Could you check a few things on this drawing? It's one solid part, dimensions in mm from its lowest x, y, z. A direction names the side the tool comes from. Give positions to 0.01 mm unless a question says otherwise; leave off trailing zeros. Order: outer loops, then holes, each group sorted by start corner. A loop starts at its lowest first (then second) coordinate and runs counter-clockwise, first axis right, second up. Notation, with made-up numbers: (52, 75.5) - (106, 75.5) arc R26 ccw to (106, 98.5) - close; hole circle Ø7 at (32.5, -26.75). An arc over 180 degrees is marked (long way). Answer as CSV lines item,"result".
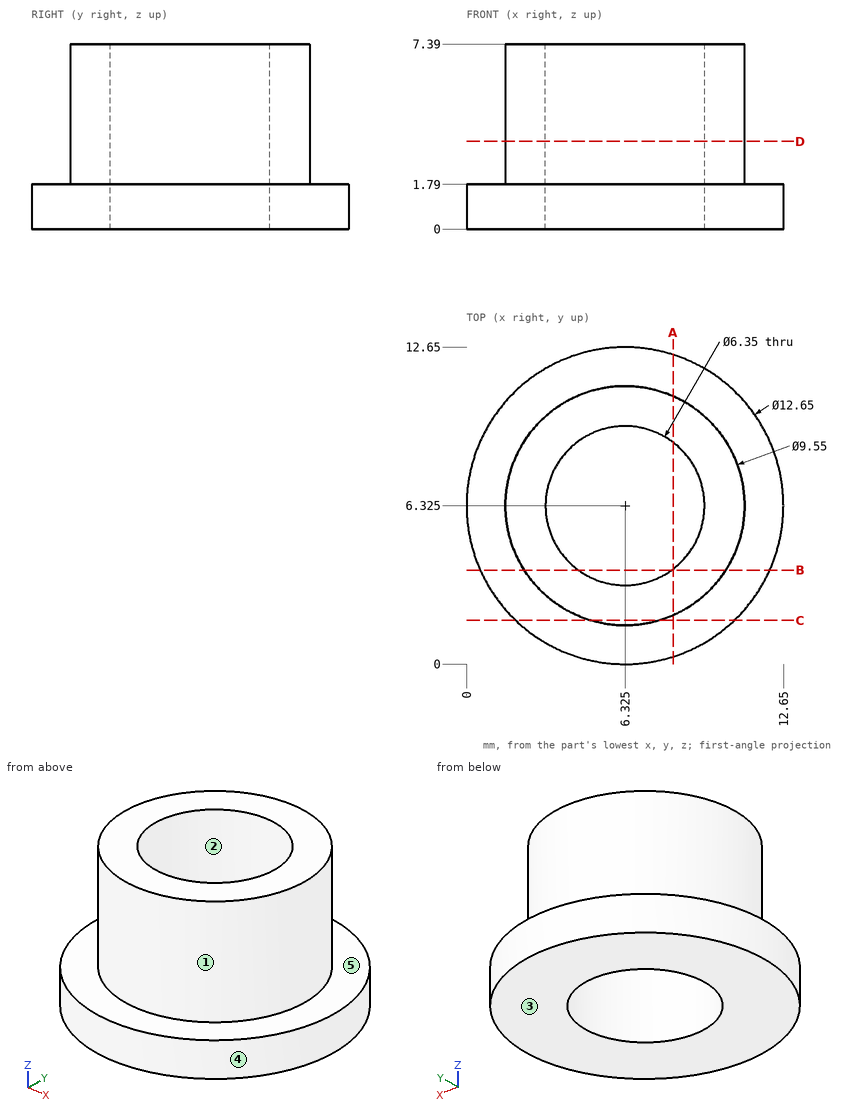
1) I'm going to push flat-ended pins straight in: P1, Ø1, axis at x = 1.5, y = 10.5, coming from the +Z side; P2, Ø6, axis at x = 2.5, y = 1.5, coming from the +Z side; P3, Ø3, axis at y = 2.5, z = 1.5, coming from the -X side; P4, Ø4, axis at y = 10, z = 6.5, coming from the +X side. Where does each tip first touch, or does it pass through?
Answer block:
P1,"z = 1.79"
P2,"z = 7.39"
P3,"x = 0.44"
P4,"x = 10.8"
2) I want a section at A-A on x = 8.25. Write out the boundary of the cut face in (y, z), plus the area to 3 significant figures.
Answer block:
outline,"(0.3, 0) - (3.8, 0) - (3.8, 7.39) - (1.96, 7.39) - (1.96, 1.79) - (0.3, 1.79) - close; (8.85, 0) - (12.35, 0) - (12.35, 1.79) - (10.69, 1.79) - (10.69, 7.39) - (8.85, 7.39) - close"
area,"33.2 mm2"
3) I want a section at D-D on z = 3.5. Write out the boundary of the cut face in (x, y) (3 decimals).
Answer block:
outline,"circle Ø9.55 at (6.325, 6.325); hole circle Ø6.35 at (6.325, 6.325)"
4) I need wall thicknesses on line 1 along Y through (x, z) = (8.5, 0.5); line 2 along Z through (x, y) = (11.75, 8.25); line 3 along Y through (x, z) = (3.75, 6.5). Which ranges of each line are inside material? Lowest first, please. Write a range as [from, to].
Answer block:
line 1,"[0.39, 4.01], [8.64, 12.26]"
line 2,"[0, 1.79]"
line 3,"[2.3, 4.47], [8.18, 10.35]"
5) I want a section at B-B on y = 3.75. Write out the boundary of the cut face in (x, z), plus the area to 3 significant figures.
Answer block:
outline,"(0.55, 0) - (4.47, 0) - (4.47, 7.39) - (2.3, 7.39) - (2.3, 1.79) - (0.55, 1.79) - close; (8.18, 0) - (12.1, 0) - (12.1, 1.79) - (10.35, 1.79) - (10.35, 7.39) - (8.18, 7.39) - close"
area,"38.3 mm2"
6) If we mould it in two halves opening along X, with no side actions, what happens to the marked faces 1, 2 and 3? For each: +X half, -X half, draft (parallel to the pull), parting line (faces both ways), or undercut.
Answer block:
face 1,"parting line"
face 2,"undercut"
face 3,"draft"
7) I want a section at C-C on y = 1.75. Write out the boundary of the cut face in (x, z).
Answer block:
outline,"(1.96, 0) - (10.69, 0) - (10.69, 1.79) - (7.69, 1.79) - (7.69, 7.39) - (4.96, 7.39) - (4.96, 1.79) - (1.96, 1.79) - close"
8) Which directions (+Z, -Z, +X, -X, +Y, -Y) give clear straight access to the entire face, cutting with the end or side of a thin tool? Please do the marked faces 4 and 5.
Answer block:
face 4,"+Z, -Z"
face 5,"+Z"
